Could you check a few things on this drawing? It's one solid part, dimensions in mm from its lowest x, y, z. Round coordinates to 2 decimals unless told otherwise and drop trailing zeros. Answer as CSV lines item,"result".
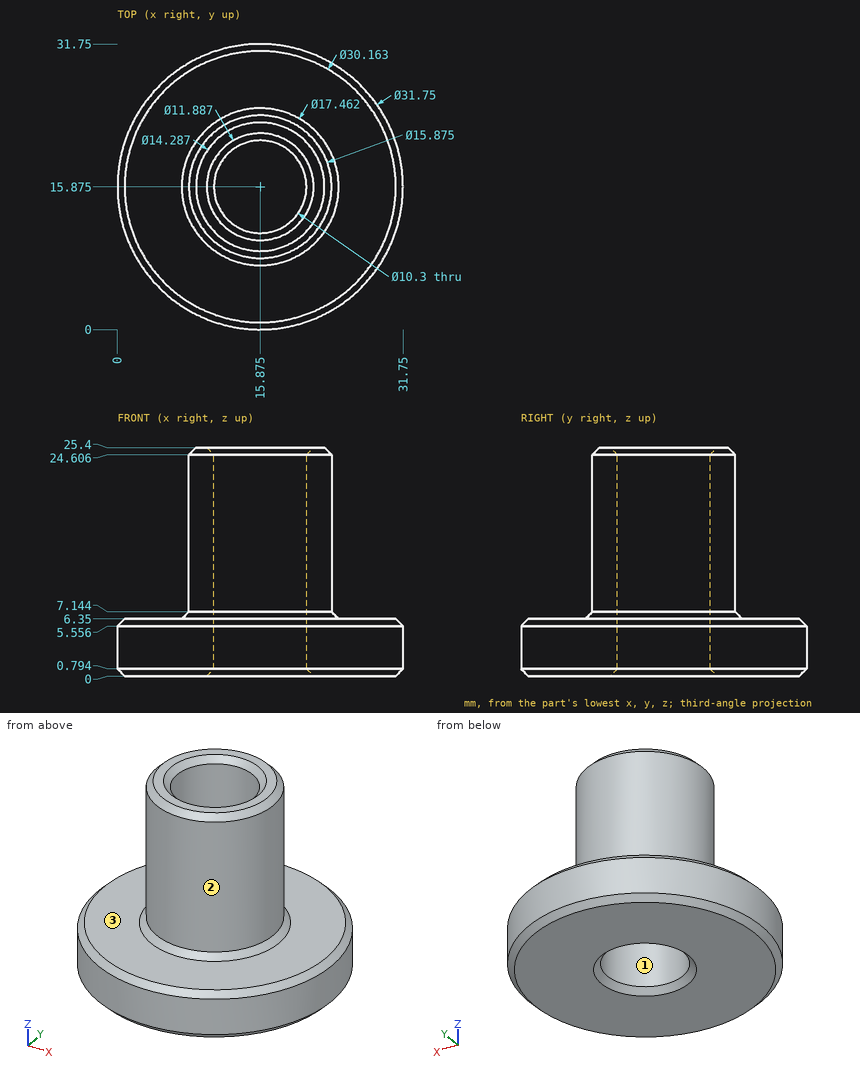
Item 1: We'd pull the mould along X, two halves only. Please class the marked faces 1, 2 and 3: released by +X, released by -X, zero draft, split by the parting line, or undercut.
Output:
face 1,"undercut"
face 2,"split by the parting line"
face 3,"zero draft"
Item 2: If I drill on line 1 along Y through (x, z) = (18, 21) (1 decimal); line 2 along X through (y, z) = (15.5, 10.5); line 3 along Y through (x, z) = (20, 1.75) (1 decimal), over which ranges is the centre line in solid material (lowest first)? Write a range as from..to.
Output:
line 1,"y = 8.2..11.2, 20.6..23.5"
line 2,"x = 7.95..10.74, 21.01..23.8"
line 3,"y = 0.5..12.8, 19..31.2"
Item 3: Will these pins go through, and if not, where does the flat tip stop? pin 1 (2 mm diameter, centred on y = 18.5, z = 21, fed in from +X) (1 decimal); pin 2 (2 mm diameter, centred on x = 7.5, y = 5.5, fed in from +Z); pin 3 (4 mm diameter, centred on x = 20.5, z = 5.5, fed in from +Y).
Output:
pin 1,"stops at x = 23.6"
pin 2,"stops at z = 6.35"
pin 3,"stops at y = 31.53"
